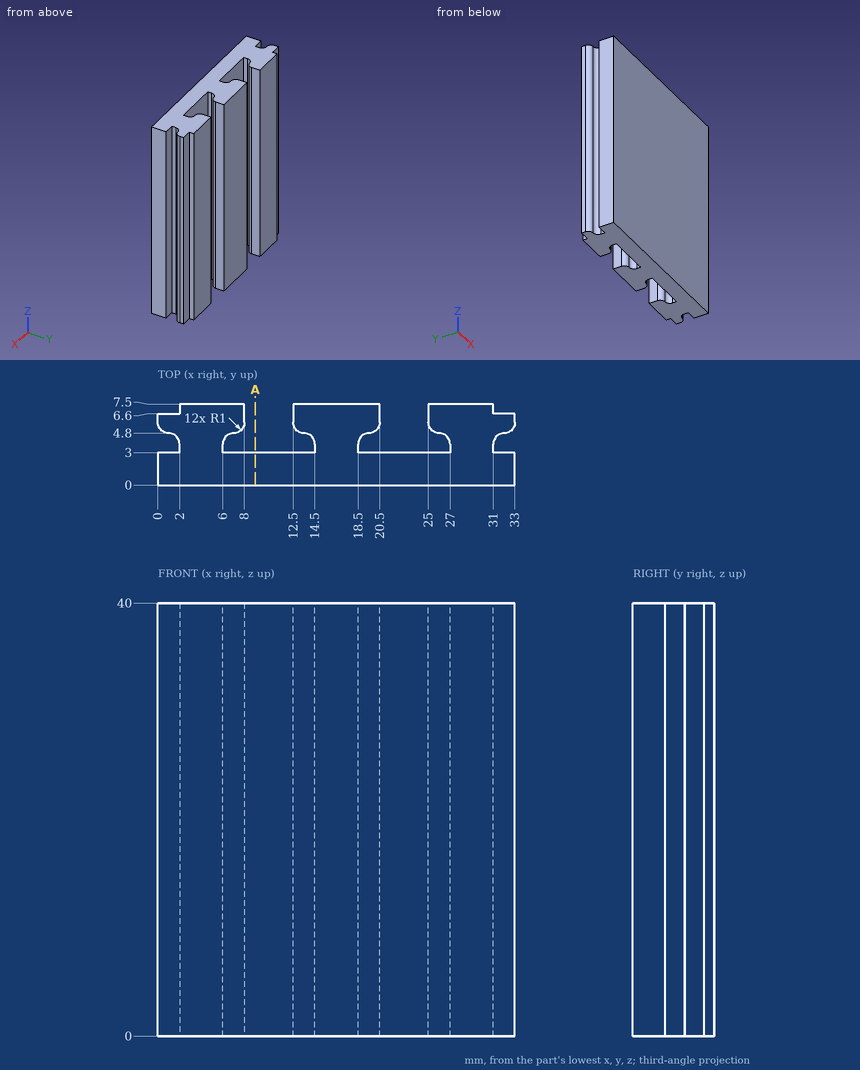
Source: three-view drawing plus pictorial views. Frame: mm from the lowest corner of the part. Give positions to 0.01 mm unless a question says otherwise; leave off trailing zeros. Order: outer loops, then holes, each group sorted by start corner. A loop starts at its lowest first (then second) coordinate and runs counter-clockwise, first axis right, second up. Notation, with made-up numbers: (70, -34.75) - (74, -34.75) arc R27 cw to (74, -12.75) - close; hole circle Ø4 at (31.5, -14.5). An arc over 180 degrees is marked (long way). Put each result on its own line as item: value.
Item 1: Ray query, L1, parallel to X at y = 6.25, z = 7; L2, parallel to X at y = 7, z = 10.5; L3, parallel to Y at x = 7, z = 26. Return the intervals inside material, ascending. Write a range as from..to.
Found:
L1: x = 0..8, 12.5..20.5, 25..33
L2: x = 2..8, 12.5..20.5, 25..31
L3: y = 0..3, 4.8..7.5
Item 2: Contact query for flat-ended pins moving along their axis: pin 1 (1.9 mm diameter, centred on y = 6.5, z = 30, fed in from -X); pin 2 (0.5 mm diameter, centred on y = 7, z = 23.5, fed in from -X); pin 3 (0.6 mm diameter, centred on y = 3.5, z = 25.5, fed in from +X). Output: stop coordinate, or through.
Found:
pin 1: stops at x = 0
pin 2: stops at x = 2
pin 3: stops at x = 31
Item 3: Section query A-A, the plane x = 9. Return loops of the section in (y, z), then the cut area to 3 significant figures.
Found:
outline: (0, 0) - (3, 0) - (3, 40) - (0, 40) - close
area: 120 mm^2
